from build123d import *

# Parameters (mm, degrees)
SKETCH2_R           = 15
BOSS_EXTRUDE2_DEPTH = 5
SKETCH3_R           = 4.5
SKETCH3_2_R         = 4.5
BOSS_EXTRUDE3_DEPTH = 6.7
SKETCH1_R           = 1
CUT_EXTRUDE1_DEPTH  = 25.225812804


with BuildPart() as part:
    # Sketch2 → Boss-Extrude2 (new body)
    with BuildSketch(Plane.XY):
        Circle(SKETCH2_R)
    extrude(amount=-BOSS_EXTRUDE2_DEPTH)

    # Sketch3 → section 0 of loft1
    with BuildSketch(Plane.XY.offset(5), mode=Mode.PRIVATE) as loft1_s0:
        Circle(SKETCH3_R)
    # loft up to a face of the part (loft1)
    loft([loft1_s0.sketch, Face(Wire([part.edges().sort_by_distance((-10.268206589, 10.934529411, 0))[0]]))])

    # Sketch3_2 → Boss-Extrude3 (add)
    with BuildSketch(Plane.XY.offset(5)):
        with Locations(Location((0, 0, 0), (0, 0, 180))):
            Circle(SKETCH3_2_R)
    extrude(amount=BOSS_EXTRUDE3_DEPTH)

    # Sketch1 → Cut-Extrude1 (cut, through all)
    with BuildSketch(Plane.XY):
        with Locations((0, 10)):
            Circle(SKETCH1_R)
        with Locations((-8.660254038, -5)):
            Circle(SKETCH1_R)
        with Locations((8.660254038, -5)):
            Circle(SKETCH1_R)
    extrude(amount=-CUT_EXTRUDE1_DEPTH, mode=Mode.SUBTRACT)


solid = part.part
The model under review builds one solid part; all positions refer to its coordinate system, in mm. A direction names the side the tool comes from. Give positions to 0.01 mm unless a question says otherwise; leave off trailing zeros. Order: outer loops, then holes, each group sorted by start corner. A loop starts at its lowest first (then second) coordinate and runs counter-clockwise, first axis right, second up. Notation, with made-up numbers: M -13,55 L 36,55 A19 ccw 36,60 Z; hole C -17,-29 d1. An arc over 180 degrees is marked long. Answer in a Markdown table with one row per item. Add a question column.
1. Add section A-A on x = 0. State the section outline as (y, z) points.
2. Machinability: for faces 4 (the flat face through (0, 10, 0)), 5 (the conical face through (4.919, 1.549, 4.687)), which of the approach directions +Z, -Z, +X, -X, +Y, -Y give a long, thin tool a straight path to every point of the face, cutting with its end or side? Answer none if there is none.
3. Mouldability with a two-part tool opening along X and no side actions: class faces 1 (the cylindrical face through (3.32, -3.04, 8.3)), 2 (the flat face through (9, -5, 0)), 3 (the flat face through (0, 0, 11.7)) as released by +X, released by -X, zero draft, split by the parting line, or undercut.
4. Add section B-B on z = -3. State the section outline as (x, y) points, plus the area to 3 significant figures.
5. To check wall thickness, follow line 1 along Y through (x, z) = (0, -1); line 2 along X through (y, z) = (8.5, -3); line 3 along X through (y, z) = (5.5, -1.25). State the ranges of each line that lie inside material, in increasing order.
6. For pin 1 Ø0.6 at (x, y) = (0, 10) entering from -Z; pin 2 Ø8 at (x, z) = (7.5, 1) entering from -Y; pin 3 Ø2 at (x, z) = (4, 6.5) entering from +Y, all flat-tipped, find the tip position at first contact; note any pin that passes through.
7. Add section C-C on z = 6.75. State the section outline as (x, y) points.
The answers:
| question | item | result |
|---|---|---|
| 1 | outline | M -15,-5 L 9,-5 L 9,0 L 11,0 L 11,-5 L 15,-5 L 15,0 L 4.5,5 L 4.5,11.7 L -4.5,11.7 L -4.5,5 L -15,0 Z |
| 2 | face 4 | -Z |
| 2 | face 5 | +Z |
| 3 | face 1 | split by the parting line |
| 3 | face 2 | undercut |
| 3 | face 3 | zero draft |
| 4 | outline | C 0,0 d30; hole C -8.66,-5 d2; hole C 0,10 d2; hole C 8.66,-5 d2 |
| 4 | area | 697 mm2 |
| 5 | line 1 | -15 to 9, 11 to 15 |
| 5 | line 2 | -12.36 to 12.36 |
| 5 | line 3 | -13.96 to 13.96 |
| 6 | pin 1 | z = 0 |
| 6 | pin 2 | y = -14.55 |
| 6 | pin 3 | y = 3.35 |
| 7 | outline | C 0,0 d9 |
